Autodesk Inventor part; units mm, degrees
ref_plane "YZ Plane" through (0, 0, 0) normal (1, 0, 0) x (0, 1, 0)
ref_plane "XZ Plane" through (0, 0, 0) normal (0, 1, 0) x (-1, 0, 0)
ref_plane "XY Plane" through (0, 0, 0) normal (0, 0, 1) x (1, 0, 0)
sketch "Sketch1" plane through (0, 0, 0) normal (0, 0, 1) x (1, 0, 0)
  circle A0 centre (0, 0) radius 14.2875
  circle A1 centre (0, 0) radius 4.7625
  circle A2 centre (0, 0) radius 15.875
  dimension "d0" = 28.575
  dimension "d1" = 9.525
  dimension "d2" = 31.75
extrude "Extrusion1" add sketch "Sketch1" along normal blind 6.3754 contours A0
extrude "Extrusion2" add sketch "Sketch1" against normal blind 1.6002 contours A0 | A2
chamfer "Chamfer1" distance 0.254 angle 45 5 edges at (-14.2875, 0, 6.3754) (-15.875, 0, 0) (-15.875, 0, -1.6002) (-4.7625, 0, 6.3754) (-4.7625, 0, -1.6002)
properties part number "fr-6-zz (1.125 OD Version)" material "Steel"
Could you check a few things on this model? Use its own coordinates, in mm. A direction names the side the tool comes from. Coordinates: 2 decimals unless noted, no trailing zeros. Write each loop counter-clockwise with the first axis right and the second up, starting at its lowest first coordinate (ties: lowest second). Pieces come first, ordered by that corner, then holes. Notation, with made-up numbers: (52, 87) -> (99, 87) arc R19 ccw to (99, 120) -> close; hole circle Ø6 at (-14, 67.25). An arc over 180 degrees is marked (long way). One line per question, with ' | ' between items. Start each with the question number.
1. If we section it at C-C (z = 1.75): Please give me the cut outline in (x, y) (1 decimal), and give its area (3 significant figures).
2. Thinking about a two-plate mould opening in X: for faces 1 (the face through (0, -6, 6.375)), 2 (the face through (-3.78, 2.9, 2.34)), 3 (the face through (-3.441, -15.497, -0.792)), which applies, pulls with the +X half, pulls with the -X half, needs draft (parallel to the pull), parting line crosses it, or undercut?
3. For faces 4 (the face through (7, -13, 0)), 5 (the face through (-4, 4, -1.6)), which set-ups out of +Z, -Z, +X, -X, +Y, -Y let a thin tool reach every point of the face, with its end or its side?
4. Please list where these lines run through material, in increasing order: line 1 along Y through (x, z) = (0, 1.75); line 2 along Z through (x, y) = (-2, 14); line 3 along X through (y, z) = (7, 6).
5. Will these pins go through, and if not, where does the flat tip stop? P1, Ø4, axis at y = -3, z = 0, coming from the +X side; P2, Ø1, axis at y = 0, z = 3.5, coming from the -X side.
Return value:
1) outline: circle Ø28.6 at (0, 0); hole circle Ø9.5 at (0, 0) | area: 570 mm²
2) face 1: needs draft | face 2: undercut | face 3: parting line crosses it
3) face 4: +Z | face 5: -Z, +X, -X, +Y, -Y
4) line 1: y = -14.29 to -4.76, 4.76 to 14.29 | line 2: z = -1.6 to 6.27 | line 3: x = -12.46 to 12.46
5) P1: stops at x = 15.84 | P2: stops at x = -14.29
